```python
from build123d import *

# Parameters (mm, degrees)
SKETCH1_R           = 1
BOSS_EXTRUDE1_DEPTH = 2
SKETCH3_R           = 1.5
SKETCH3_W           = 10
SKETCH3_H           = 10
BOSS_EXTRUDE2_DEPTH = 8.4
SKETCH5_W           = 10.532166359
SKETCH5_H           = 2
BOSS_EXTRUDE3_DEPTH = 13
SKETCH6_W           = 10
SKETCH6_H           = 4
SKETCH6_W_2         = 13.935667282
SKETCH6_H_2         = 6.95
SKETCH6_W_3         = 7
SKETCH6_H_3         = 6
BOSS_EXTRUDE4_DEPTH = 2
SKETCH7_W           = 3
SKETCH7_H           = 8
SKETCH7_W_2         = 2
SKETCH7_H_2         = 12
BOSS_EXTRUDE5_DEPTH = 6
SKETCH8_W           = 2
SKETCH8_H           = 14
BOSS_EXTRUDE6_DEPTH = 8
BOSS_EXTRUDE7_DEPTH = 15


with BuildPart() as part:
    # Sketch1 → Boss-Extrude1 (new body)
    with BuildSketch(Plane.XY):
        Polygon((90.25, -53.25), (-72.25, -53.25), (-72.25, 53.25), (70.25, 53.25), (90.25, 33.25), align=None)
        with Locations((3.75, -8.25)):
            Circle(SKETCH1_R, mode=Mode.SUBTRACT)
        with Locations((26.25, -8.25)):
            Circle(SKETCH1_R, mode=Mode.SUBTRACT)
        with Locations((26.25, 48.75)):
            Circle(SKETCH1_R, mode=Mode.SUBTRACT)
        with Locations((3.75, 48.75)):
            Circle(SKETCH1_R, mode=Mode.SUBTRACT)
    extrude(amount=-BOSS_EXTRUDE1_DEPTH)

    # Sketch3 → Boss-Extrude2 (add)
    # profile 1 of 4: a face of its own
    with BuildSketch(Plane.XY):
        Polygon((61.75, 52.75), (70.75, 52.75), (71.75, 51.75), (71.75, 42.75), (61.75, 42.75), align=None)
        with Locations((66.75, 47.75)):
            Circle(SKETCH3_R, mode=Mode.SUBTRACT)
    # profile 2 of 4: a face of its own
    with BuildSketch(Plane.XY):
        with Locations((66.75, -47.75)):
            Rectangle(SKETCH3_W, SKETCH3_H)
        with Locations((66.75, -47.75)):
            Circle(SKETCH3_R, mode=Mode.SUBTRACT)
    # profile 3 of 4: a face of its own
    with BuildSketch(Plane.XY):
        with Locations((-66.75, 47.75)):
            Rectangle(SKETCH3_W, SKETCH3_H)
        with Locations((-66.75, 47.75)):
            Circle(SKETCH3_R, mode=Mode.SUBTRACT)
    # profile 4 of 4: a face of its own
    with BuildSketch(Plane.XY):
        with Locations((-66.75, -47.75)):
            Rectangle(SKETCH3_W, SKETCH3_H)
        with Locations((-66.75, -47.75)):
            Circle(SKETCH3_R, mode=Mode.SUBTRACT)
    extrude(amount=BOSS_EXTRUDE2_DEPTH)

    # Sketch5 → Boss-Extrude3 (add)
    with BuildSketch(Plane.XY):
        Polygon((90.25, 33.25), (90.25, -53.25), (-72.25, -53.25), (-72.25, 53.25), (-12.75, 53.25), (-12.75, 51.25), (-70.25, 51.25), (-70.25, -51.25), (88.25, -51.25), (88.25, 32.421572875), (69.421572875, 51.25), (39.25, 51.25), (39.25, 53.25), (70.25, 53.25), align=None)
        with Locations((2.51608318, 52.25)):
            Rectangle(SKETCH5_W, SKETCH5_H)
        with Locations((26.98391682, 52.25)):
            Rectangle(SKETCH5_W, SKETCH5_H)
    extrude(amount=BOSS_EXTRUDE3_DEPTH)

    # Sketch6 → Boss-Extrude4 (add)
    with BuildSketch(Plane(origin=(0, 53.25, 0), x_dir=(1, 0, 0), z_dir=(0, 1, 0))):
        with Locations((-7.75, -11)):
            Rectangle(SKETCH6_W, SKETCH6_H)
        with Locations((14.75, -9.525)):
            Rectangle(SKETCH6_W_2, SKETCH6_H_2)
        with Locations((35.75, -10)):
            Rectangle(SKETCH6_W_3, SKETCH6_H_3)
    extrude(amount=-BOSS_EXTRUDE4_DEPTH)

    # Sketch7 → Boss-Extrude5 (add)
    with BuildSketch(Plane.XY):
        with Locations((35.75, 37.25)):
            Rectangle(SKETCH7_W, SKETCH7_H)
        with Locations((31.25, 39.25)):
            Rectangle(SKETCH7_W_2, SKETCH7_H_2)
        with Locations((40.25, 39.25)):
            Rectangle(SKETCH7_W_2, SKETCH7_H_2)
    extrude(amount=BOSS_EXTRUDE5_DEPTH)

    # Sketch8 → Boss-Extrude6 (add)
    with BuildSketch(Plane.XY):
        with Locations((-13.75, 33.25)):
            Rectangle(SKETCH8_W, SKETCH8_H)
        Polygon((-7.75, 26.25), (-7.75, 32.25), (-3.75, 32.25), (-2.75, 32.25), (-2.75, 40.25), (-0.75, 40.25), (-0.75, 26.25), (-2.75, 26.25), align=None)
    extrude(amount=BOSS_EXTRUDE6_DEPTH)

    # Sketch9 → Boss-Extrude7 (add)
    with BuildSketch(Plane(origin=(0, 0, -2), x_dir=(-1, 0, 0), z_dir=(0, 0, -1))):
        Polygon((-92.25, 7.5), (-90.25, 7.5), (-90.25, 9.5), (-90.25, 13.5), (-94.25, 9.5), (-94.25, -9.5), (-90.25, -13.5), (-90.25, -9.5), (-90.25, -7.5), (-92.25, -7.5), align=None)
    extrude(amount=-BOSS_EXTRUDE7_DEPTH)


solid = part.part
```
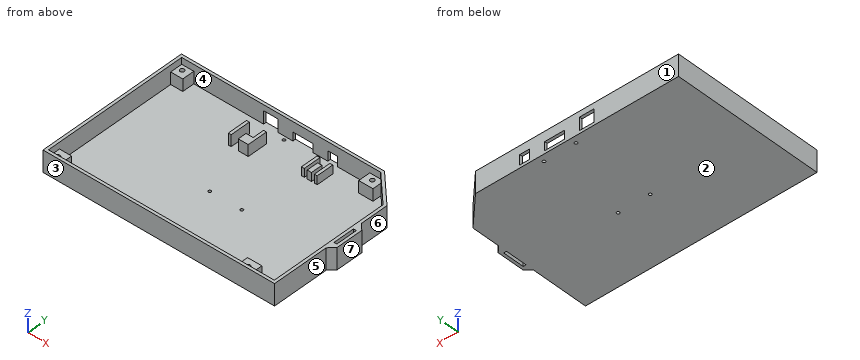
Part model, mm, in its own coordinate system. Face numbers are marked on the shaded views. A direction names the side the tool comes from. Give positions to 0.01 mm unless a question says otherwise; leave off trailing zeros. Write each loop counter-clockwise with the first axis right and the second up, starting at its lowest first coordinate (ties: lowest second). Pieces come first, ordered by that corner, then holes. Notation, with made-up numbers: M 3,17.5 L 45,17.5 A20 cw 45,50.5 Z; hole C 51.5,-14.75 d4. An arc over 180 degrees is marked long. Use CSV: the item, a comma, the result in double quotes.
Item 1: Drill centre lines: probe 1 along X at (y, z) = (6, 4); probe 2 along X at (y, z) = (26.5, 7.5); probe 3 along Y at (x, z) = (3.75, -0.5). Where is each one in solid material? Low to high.
Taken from the geometry:
probe 1,"x = -72.25 to -70.25, 88.25 to 90.25, 92.25 to 94.25"
probe 2,"x = -72.25 to -70.25, -14.75 to -12.75, -7.75 to -0.75, 88.25 to 90.25"
probe 3,"y = -53.25 to -9.25, -7.25 to 47.75, 49.75 to 53.25"
Item 2: Slice it at B-B on y = -31.5. Write the cut outline in (x, z), plus the area to 3 significant figures.
Taken from the geometry:
outline,"M -72.25,-2 L 90.25,-2 L 90.25,13 L 88.25,13 L 88.25,0 L -70.25,0 L -70.25,13 L -72.25,13 Z"
area,"377 mm²"
Item 3: Pull direction Y, two halves, no side cores. Call the marked faces 1, 2, 3 and 4: +Y half, -Y half, draft (parallel to the pull), parting line (faces both ways), or undercut.
Taken from the geometry:
face 1,"+Y half"
face 2,"draft"
face 3,"-Y half"
face 4,"undercut"
Item 4: Pin check, flat tips, straight feed: P1, Ø6.5, axis at y = 38, z = 3, coming from the +X side; P2, Ø0.9, axis at x = -67, y = 48, coming from the +Z side; P3, Ø2.5, axis at y = -46, z = 2.5, coming from the +X side. Stop position of each tip, or through.
Taken from the geometry:
P1,"stops at x = 88.75"
P2,"stops at z = 0"
P3,"stops at x = 90.25"
Item 5: Slice it at A-A on x = 16. Write the cut outline in (y, z).
Taken from the geometry:
outline,"M -53.25,-2 L 53.25,-2 L 53.25,0 L -51.25,0 L -51.25,13 L -53.25,13 Z; M 51.25,6.05 L 53.25,6.05 L 53.25,13 L 51.25,13 Z"
Item 6: Which spindle directions (+Z, -Z, +X, -X, +Y, -Y) get a long thin tool onto all of the face, cutting with end or side? Do the marked faces 5, 6 and 7. Say none if no direction does.
Taken from the geometry:
face 5,"+Z, -Z, +X, -Y"
face 6,"+Z, -Z, +X, +Y"
face 7,"+Z, -Z, +X, +Y, -Y"
